Source: CAD feature listing. Evaluate the final solid. Frame: model axes, mm. Face numbers are marked on the shaded views. A direction names the side the tool comes from. Round coordinates to 2 decimals unless told otherwise and drop trailing zeros. Order: outer loops, then holes, each group sorted by start corner. A loop starts at its lowest first (then second) coordinate and runs counter-clockwise, first axis right, second up. Notation, with made-up numbers: (81.25, 55.25) -> (98.25, 55.25) arc R16 cw to (98.25, 65.25) -> close; hole circle Ø7 at (-10, -32.75). An arc over 180 degrees is marked (long way). Write item = value, one per line. Start each with the question number.
(1) Contact query for flat-ended pins moving along their axis: pin 1 Ø18.5 at (x, z) = (-34.5, 25) entering from -Y; pin 2 Ø6 at (x, z) = (-21.5, 28) entering from -Y; pin 3 Ø5.5 at (y, z) = (8, 1.5) entering from +X; pin 4 Ø3 at (x, y) = (-15.4, 25.8) entering from -Z. Output: stop coordinate, or through.
(2) Cut plane D-D on y = 66. Return the cut outline in (x, z).
(3) Cut plane B-B on y = -25.8. Return the cut outline in (x, z), then the cut area to 3 significant figures.
(4) Cut plane C-C on z = 28.5. Return the cut outline in (x, y).
(5) Reachability of the marked faces 1, 2 and 3 from +Z, -Z, +X, -X, +Y, -Y: full face, straight path, thin tool, end or side. Return the list, or none.
(6) Cut plane A-A on x = -15.4. Return the cut outline in (y, z).
(7) Draft query along Y for the marked faces 4, 5 and 6. Return one class per face: released by +Y, released by -Y, zero draft, split by the parting line, or undercut.
(8) Ray query, line 1 (Y direction, x = -4.6, z = 1.6); line 2 (X direction, y = 25, z = 3); line 3 (X direction, y = 25, z = 2). Return the intervals inside material, ascending.
from build123d import *

# Parameters (mm, degrees)
ESQUISSE1_W             = 40
ESQUISSE1_H             = 60
ESQUISSE1_W_2           = 20.6
ESQUISSE1_H_2           = 40.6
BOSS_EXTRU_1_DEPTH      = 5
ESQUISSE2_W             = 40
ESQUISSE2_H             = 5
BOSS_EXTRU_2_DEPTH      = 26
BOSS_EXTRU_5_DEPTH      = 40
BOSS_EXTRU_6_DEPTH      = 26
CONG_1_R                = 13
CONG_2_R                = 4
ENL_V_MAT_EXTRU_1_REACH = 141.98
ESQUISSE6_R             = 2.5


with BuildPart() as part:
    # Esquisse1 → Boss.-Extru.1 (new body)
    with BuildSketch(Plane.XY):
        with Locations((-10, 0)):
            Rectangle(ESQUISSE1_W, ESQUISSE1_H)
        with Locations((-10, 0)):
            Rectangle(ESQUISSE1_W_2, ESQUISSE1_H_2, mode=Mode.SUBTRACT)
    extrude(amount=BOSS_EXTRU_1_DEPTH)

    # Esquisse2 → Boss.-Extru.2 (add)
    with BuildSketch(Plane(origin=(0, 30, 0), x_dir=(1, 0, 0), z_dir=(0, 1, 0))):
        with Locations((-10, -2.5)):
            Rectangle(ESQUISSE2_W, ESQUISSE2_H)
    extrude(amount=BOSS_EXTRU_2_DEPTH)

    # Esquisse3 → Boss.-Extru.5 (add)
    with BuildSketch(Plane(origin=(10, 0, 0), x_dir=(0, 0, -1), z_dir=(1, 0, 0))):
        Polygon((0, 56), (-70, 105.014527675), (-70, 101.513489984), (-5, 56), align=None)
        Polygon((-5, -30), (0, -30), (-70, -62.641536071), (-70, -60.30999778), align=None)
    extrude(amount=-BOSS_EXTRU_5_DEPTH)

    # Esquisse4 → Boss.-Extru.6 (add)
    with BuildSketch(Plane(origin=(0, 0, 0), x_dir=(1, 0, 0), z_dir=(0, 1, 0))):
        Polygon((-30, -5), (-58.368325731, -70), (-60.550504633, -70), (-30, 0), align=None)
        Polygon((10, 0), (40.550504633, -70), (38.368325731, -70), (10, -5), align=None)
    extrude(amount=BOSS_EXTRU_6_DEPTH)

    # Congé1
    cong_1_edges = [part.edges().sort_by_distance(p)[0] for p in [
        (-10, 56, 5),
        (10, 13, 5),
        (-30, 13, 5),
    ]]
    fillet(cong_1_edges, radius=CONG_1_R)

    # Congé2
    cong_2_edges = [part.edges().sort_by_distance(p)[0] for p in [
        (10, 103.264008829, 70),
        (-30, 103.264008829, 70),
        (10, -61.475766925, 70),
        (-30, -61.475766925, 70),
        (-59.459415182, 0, 70),
        (-59.459415182, 26, 70),
        (39.459415182, 0, 70),
        (39.459415182, 26, 70),
    ]]
    fillet(cong_2_edges, radius=CONG_2_R)

    # Esquisse6 → Enlèv. mat.-Extru.1 (cut, up to next)
    with BuildSketch(Plane(origin=(0, 0, 0), x_dir=(-1, 0, 0), z_dir=(0, 0, -1)), mode=Mode.PRIVATE) as enl_v_mat_extru_1_sk1:
        with Locations((4.6, -25.8)):
            Circle(ESQUISSE6_R)
    enl_v_mat_extru_1_tool1 = extrude(enl_v_mat_extru_1_sk1.sketch, amount=-ENL_V_MAT_EXTRU_1_REACH, mode=Mode.PRIVATE) & part.part
    # Esquisse6 → Enlèv. mat.-Extru.1 (cut, up to next)
    with BuildSketch(Plane(origin=(0, 0, 0), x_dir=(-1, 0, 0), z_dir=(0, 0, -1)), mode=Mode.PRIVATE) as enl_v_mat_extru_1_sk2:
        with Locations((15.4, -25.8)):
            Circle(ESQUISSE6_R)
    enl_v_mat_extru_1_tool2 = extrude(enl_v_mat_extru_1_sk2.sketch, amount=-ENL_V_MAT_EXTRU_1_REACH, mode=Mode.PRIVATE) & part.part
    # Esquisse6 → Enlèv. mat.-Extru.1 (cut, up to next)
    with BuildSketch(Plane(origin=(0, 0, 0), x_dir=(-1, 0, 0), z_dir=(0, 0, -1)), mode=Mode.PRIVATE) as enl_v_mat_extru_1_sk3:
        with Locations((4.6, 25.8)):
            Circle(ESQUISSE6_R)
    enl_v_mat_extru_1_tool3 = extrude(enl_v_mat_extru_1_sk3.sketch, amount=-ENL_V_MAT_EXTRU_1_REACH, mode=Mode.PRIVATE) & part.part
    # Esquisse6 → Enlèv. mat.-Extru.1 (cut, up to next)
    with BuildSketch(Plane(origin=(0, 0, 0), x_dir=(-1, 0, 0), z_dir=(0, 0, -1)), mode=Mode.PRIVATE) as enl_v_mat_extru_1_sk4:
        with Locations((15.4, 25.8)):
            Circle(ESQUISSE6_R)
    enl_v_mat_extru_1_tool4 = extrude(enl_v_mat_extru_1_sk4.sketch, amount=-ENL_V_MAT_EXTRU_1_REACH, mode=Mode.PRIVATE) & part.part
    add(enl_v_mat_extru_1_tool1.solids().sort_by_distance((-4.6, -25.8, 0))[0], mode=Mode.SUBTRACT)
    add(enl_v_mat_extru_1_tool2.solids().sort_by_distance((-15.4, -25.8, 0))[0], mode=Mode.SUBTRACT)
    add(enl_v_mat_extru_1_tool3.solids().sort_by_distance((-4.6, 25.8, 0))[0], mode=Mode.SUBTRACT)
    add(enl_v_mat_extru_1_tool4.solids().sort_by_distance((-15.4, 25.8, 0))[0], mode=Mode.SUBTRACT)


solid = part.part
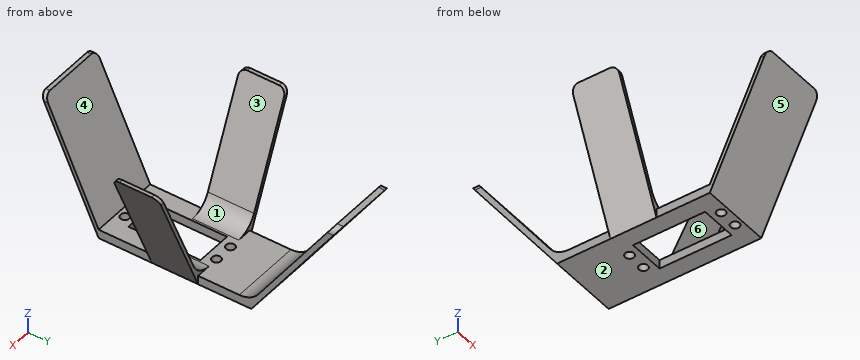
Evaluation:
q1.pin_1 = -45.43
q1.pin_2 = -44.46
q1.pin_3 = 11.85
q1.pin_4 = through
q2.outline = (-30, 14.28) -> (10, 14.28) -> (10, 19.28) -> (-30, 19.28) -> close
q3.outline = (-30, 0) -> (-17.9, 0) -> (-17.9, 5) -> (-30, 5) -> close; (-12.9, 0) -> (-7.1, 0) -> (-7.1, 5) -> (-12.9, 5) -> close; (-2.1, 0) -> (10, 0) -> (10, 5) -> (-2.1, 5) -> close
q3.area = 150 mm^2
q4.outline = (-42.44, 0) -> (-40.26, 0) -> (-40.26, 26) -> (-42.44, 26) -> close; (-30, -43.29) -> (10, -43.29) -> (10, -40.96) -> (-30, -40.96) -> close; (-30, 72.45) -> (10, 72.45) -> (10, 75.96) -> (-30, 75.96) -> close; (20.26, 0) -> (22.44, 0) -> (22.44, 26) -> (20.26, 26) -> close
q5.face_1 = +Z
q5.face_2 = -Z, +X, -X, +Y, -Y
q5.face_3 = +Z, +Y, -Y
q6.outline = (-62.64, 70) -> (-30, 0) -> (-28.3, 0) -> (-28.3, 5) -> (-30, 5) -> (-60.31, 70) -> close; (-23.3, 0) -> (-20.3, 0) -> (-20.3, 5) -> (-23.3, 5) -> close; (20.3, 0) -> (23.3, 0) -> (23.3, 5) -> (20.3, 5) -> close; (28.3, 0) -> (56, 0) -> (105.01, 70) -> (101.51, 70) -> (59.88, 10.54) arc R13 cw to (49.23, 5) -> (28.3, 5) -> close
q7.face_4 = undercut
q7.face_5 = released by -Y
q7.face_6 = zero draft
q8.line_1 = -30.75 to -28.3, -23.3 to -20.3, 20.3 to 23.3, 28.3 to 57.12
q8.line_2 = -31.31 to -17.77, -13.03 to -6.97, -2.23 to 11.31
q8.line_3 = -30.87 to -17.77, -13.03 to -6.97, -2.23 to 10.87
